Check sheet for the modelled part. Datum: model origin and axes. Units: mm. A direction names the side the tool comes from. Round coordinates to 2 decimals unless told otherwise and drop trailing zeros. Write each loop counter-clockwise with the first axis right and the second up, starting at its lowest first coordinate (ties: lowest second). Pieces come first, ordered by that corner, then holes. Notation, with made-up numbers: (-37, 73) -> (-20, 73) arc R21 ccw to (-20, 80) -> close; hole circle Ø1 at (71.25, 28). An arc over 180 degrees is marked (long way). Put each result on its own line as item: value. Start each with the question number.
Autodesk Fusion 360 part; units mm, degrees
sketch "草图1" plane through (0, 0, 0) normal (0, 0, 1) x (1, 0, 0)
  line L0 (15, -10) -> (-15, -10)
  line L1 (-15, -10) -> (-15, 10)
  line L2 (-15, 10) -> (15, 10)
  line L3 (15, 10) -> (15, -10)
  line L4 (15, -10) -> (-15, 10) construction
  line L5 (-15, -10) -> (15, 10) construction
  line L6 (0, 0) -> (19, 0) construction
  line L7 (0, 0) -> (9.0277, 9.0277) construction
  circle A0 centre (0, 0) radius 7 construction
  circle A1 centre (4.9497, 4.9497) radius 1.75
  circle A2 centre (-4.9497, 4.9497) radius 1.75
  circle A3 centre (-4.9497, -4.9497) radius 1.75
  circle A4 centre (4.9497, -4.9497) radius 1.75
  circle A5 centre (0, 0) radius 3
  dimension "d1" = 20
  dimension "d2" = 30
  dimension "d3" = 45
  dimension "d4" = 14
  dimension "d5" = 3.5
  dimension "d7" = 360
  dimension "d8" = 6
extrude "拉伸1" add sketch "草图1" along normal blind 6 makes body 1
sketch "草图2" plane through (0, 0, 0) normal (0, 0, -1) x (1, 0, 0)
  circle A0 centre (0, 0) radius 3
  circle A1 centre (4.9497, -4.9497) radius 1.75
  circle A2 centre (-4.9497, 4.9497) radius 1.75
  circle A3 centre (4.9497, 4.9497) radius 1.75
  circle A4 centre (-4.9497, -4.9497) radius 1.75
  line L0 (-15, -10) -> (15, -10)
  line L1 (15, -10) -> (15, 10)
  line L2 (15, 10) -> (-15, 10)
  line L3 (-15, 10) -> (-15, -10)
  line L4 (15, -10) -> (10, -10)
  line L5 (10, -10) -> (10, 10)
  line L6 (10, 10) -> (15, 10)
  line L7 (15, 10) -> (15, -10)
  line L8 (-15, -10) -> (-10, -10)
  line L9 (-10, -10) -> (-10, 10)
  line L10 (-10, 10) -> (-15, 10)
  line L11 (-15, 10) -> (-15, -10)
  dimension "d11" = 5
  dimension "d12" = 5
extrude "拉伸2" add sketch "草图2" along normal blind 100 contours L0 L2 L3 L8 L9 L10 L11 | L0 L1 L2 L4 L5 L6 L7 bodies 1
sketch "草图3" plane through (0, 0, -100) normal (0, 0, -1) x (1, 0, 0)
  line L0 (-15, 10) -> (-15, -10)
  line L1 (-15, -10) -> (-10, -10)
  line L2 (-10, -10) -> (-10, 10)
  line L3 (-10, 10) -> (-15, 10)
  line L4 (-10, 10) -> (-10, -10)
  line L5 (-10, -10) -> (10, -10)
  line L6 (10, -10) -> (10, 10)
  line L7 (10, 10) -> (-10, 10)
  circle A0 centre (-4.9497, -4.9497) radius 1.75
  circle A1 centre (4.9497, 4.9497) radius 1.75
  circle A2 centre (-4.9497, 4.9497) radius 1.75
  circle A3 centre (4.9497, -4.9497) radius 1.75
  circle A4 centre (0, 0) radius 3
  line L8 (15, 10) -> (10, 10)
  line L9 (10, 10) -> (10, -10)
  line L10 (10, -10) -> (15, -10)
  line L11 (15, -10) -> (15, 10)
extrude "拉伸3" add sketch "草图3" along normal blind 6 bodies 1
sketch "草图4" plane through (0, 10, 0) normal (0, 1, 0) x (-1, 0, 0)
  line L0 (15, -106) -> (15, 6)
  line L1 (15, 6) -> (-15, 6)
  line L2 (-15, 6) -> (-15, -106)
  line L3 (-15, -106) -> (15, -106)
  line L4 (10, -100) -> (-10, -100)
  line L5 (-10, -100) -> (-10, 0)
  line L6 (-10, 0) -> (10, 0)
  line L7 (10, 0) -> (10, -100)
  line L8 (47.9011, -50) -> (-70, -50)
  line L9 (0, -112.7701) -> (0, 40) construction
  line L10 (-10, -63.5355) -> (-13.5355, -60)
  line L11 (-13.5355, -60) -> (10, -36.4645)
  line L12 (10, -36.4645) -> (13.5355, -40)
  line L13 (13.5355, -40) -> (-10, -63.5355)
  line L14 (-10, -63.5355) -> (10, -36.4645)
  line L15 (13.5355, -40) -> (-13.5355, -60)
  line L16 (-10, -36.4645) -> (-13.5355, -40)
  line L17 (13.5355, -60) -> (-10, -36.4645)
  line L18 (-13.5355, -40) -> (10, -63.5355)
  line L19 (10, -63.5355) -> (13.5355, -60)
  line L20 (-10, -36.4645) -> (10, -63.5355)
  line L21 (13.5355, -60) -> (-13.5355, -40)
  point P0 (0, -50)
  dimension "d17" = 45
  dimension "d18" = 5
extrude "拉伸4" add sketch "草图4" against normal blind 20 contours L7 L13 L15 L17 | L7 L13 L17 L21 | L8 L13 L21 | L8 L15 L17 | L7 L14 L15 L17 | L7 L13 L20 L21 | L8 L15 L18 | L13 L14 L18 L20 | L11 L14 L17 L20 | L14 L15 L17 | L14 L15 L18 | L11 L20 L21 | L13 L20 L21 | L8 L11 L21 | L5 L11 L15 L18 | L5 L11 L18 L21 | L11 L14 L17 | L13 L18 L20 | L13 L14 L18 | L5 L14 L15 L18 | L11 L17 L20 | L5 L11 L20 L21 bodies 1
sketch "草图5" plane through (0, 0, -106) normal (0, 0, -1) x (1, 0, 0)
  circle A0 centre (4.9497, -4.9497) radius 1.75
  circle A1 centre (4.9497, 4.9497) radius 1.75
  circle A2 centre (-4.9497, 4.9497) radius 1.75
  circle A3 centre (0, 0) radius 3
  circle A4 centre (-4.9497, -4.9497) radius 1.75
  line L0 (15, -10) -> (15, 10)
  line L1 (15, 10) -> (-10, 10)
  line L2 (-10, 10) -> (-15, 10)
  line L3 (-15, 10) -> (-15, -10)
  line L4 (-15, -10) -> (15, -10)
  circle A5 centre (0, 0) radius 3
extrude "拉伸5" cut sketch "草图5" against normal blind 112 contours A3 A5 bodies 1
copy_body "实体->零部件1" bodies 1 removing the originals makes body 2 in component "Component'"
component "Component'" placed x (1, 0, 0) y (0, 1, 0) z (0, 0, 1) at (0, 0, 0)
1. Material ranges on L1, parallel to Z at x = -3, y = -9; L2, parallel to Y at x = 0, z = 3.5; L3, parallel to Z at x = -7, y = 0.25, recorded low to high. Write a range as [from, to].
2. Section check B-B, the plane z = -28.5. Enter the section's corners in (x, y), then the cut area to 3 significant figures.
3. Section check A-A, the plane y = 0. Give the number of separate pieces and of enclosed holes in the cut face, then the cut area to 3 significant figures.
4. Draft check along X on faces 1 (the flat face through (15, 0, -51)), 2 (the flat face through (-4, 0, -106)), 3 (the cylindrical face through (-4.14, 3.4, -102.96)). Enter one of: released by +X, released by -X, zero draft, split by the parting line, or undercut.
5. Access from +Z, -Z, +X, -X, +Y, -Y to the whole of each face (thin tool, end or side, straight path). Record for faces 4 (the flat face through (-2.4, 2.4, 0)), 5 (the cylindrical face through (-4.14, 6.5, 2.96)), 6 (the cylindrical face through (-4.14, -6.5, -102.96)), 7 (the flat face through (-4, 0, 6)).
6. Gauge pin test, flat ends, axial feed: P1, Ø4.5, axis at x = -4.95, y = 4.95, coming from the -Z side; P2, Ø3, axis at x = 4.95, y = -4.95, coming from the +Z side; P3, Ø3, axis at x = 4.95, y = 4.95, coming from the -Z side. Record the tip position at first contact, or that the pin passes through.
Reply:
1. L1: z = [-106, -100], [-56.54, -43.46], [0, 6]
1. L2: y = [-10, -3], [3, 10]
1. L3: z = [-106, -100], [-60.54, -53.46], [-46.54, -39.46], [0, 6]
2. outline: (-15, -10) -> (-10, -10) -> (-10, 10) -> (-15, 10) -> close; (10, -10) -> (15, -10) -> (15, 10) -> (10, 10) -> close
2. area: 200 mm2
3. separate pieces: 2
3. enclosed holes: 2
3. area: 1,490 mm2
4. face 1: released by +X
4. face 2: zero draft
4. face 3: undercut
5. face 4: +Y, -Y
5. face 5: +Z
5. face 6: -Z
5. face 7: +Z, +X, -X, +Y, -Y
6. P1: stops at z = -106
6. P2: stops at z = -40.01
6. P3: stops at z = -59.99
